from build123d import *

# Parameters (mm, degrees)
CROQUIS1_R              = 1.35
SALIENTE_EXTRUIR1_DEPTH = 10
CROQUIS2_W              = 7
CROQUIS2_H              = 28
SALIENTE_EXTRUIR2_DEPTH = 20
CROQUIS3_R              = 1.35
CORTAR_EXTRUIR1_DEPTH   = 15


with BuildPart() as part:
    # Croquis1 → Saliente-Extruir1 (new body)
    with BuildSketch(Plane(origin=(0, 0, 0), x_dir=(1, 0, 0), z_dir=(0, 1, 0))):
        Polygon((-20.25, -20), (-20.25, 8), (20.25, 8), (20.25, -20), (27.25, -20), (27.25, 20), (-27.25, 20), (-27.25, -20), align=None)
        with Locations(Location((-20.25, 15, 0), (0, 0, 270))):
            Circle(CROQUIS1_R, mode=Mode.SUBTRACT)
        with Locations(Location((20.25, 15, 0), (0, 0, 90))):
            Circle(CROQUIS1_R, mode=Mode.SUBTRACT)
    extrude(amount=SALIENTE_EXTRUIR1_DEPTH)

    # Croquis2 → Saliente-Extruir2 (add)
    with BuildSketch(Plane(origin=(0, 0, 0), x_dir=(1, 0, 0), z_dir=(0, 1, 0))):
        with Locations((-23.75, -6)):
            Rectangle(CROQUIS2_W, CROQUIS2_H)
        with Locations((23.75, -6)):
            Rectangle(CROQUIS2_W, CROQUIS2_H)
    extrude(amount=SALIENTE_EXTRUIR2_DEPTH)

    # Croquis3 → Cortar-Extruir1 (cut)
    with BuildSketch(Plane.XY.offset(20)):
        with Locations((-24.75, 15.612517806)):
            Circle(CROQUIS3_R)
        with Locations((-24.75, 4.5)):
            Circle(CROQUIS3_R)
        with Locations(Location((24.75, 4.5, 0), (0, 0, 180))):
            Circle(CROQUIS3_R)
        with Locations(Location((24.75, 15.612517806, 0), (0, 0, 180))):
            Circle(CROQUIS3_R)
    extrude(amount=-CORTAR_EXTRUIR1_DEPTH, mode=Mode.SUBTRACT)


solid = part.part
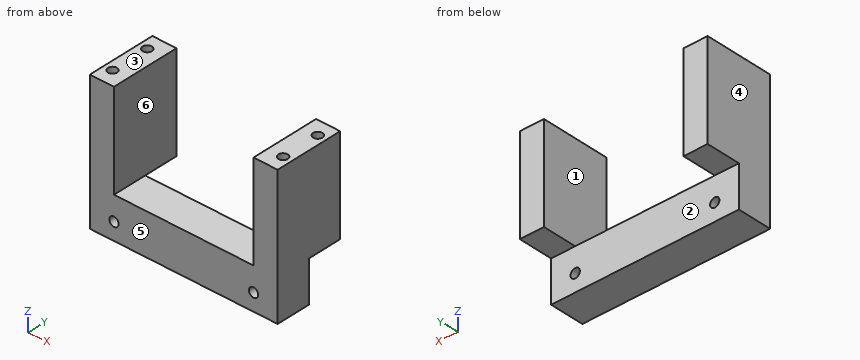
Build history of the part. All positions in model axes, mm. Face numbers are marked on the shaded views. A direction names the side the tool comes from. Coordinates: 2 decimals unless noted, no trailing zeros. Order: outer loops, then holes, each group sorted by start corner. A loop starts at its lowest first (then second) coordinate and runs counter-clockwise, first axis right, second up. Notation, with made-up numbers: (-38, 51) - (4, 51) arc R25 cw to (4, 77) - close; hole circle Ø2 at (18, 20.5). An arc over 180 degrees is marked (long way). Put each result on its own line as item: value.
1. Pull direction X, two halves, no side cores. Call the marked faces 4, 5 and 6: pulls with the +X half, pulls with the -X half, needs draft (parallel to the pull), parting line crosses it, or undercut.
Answer sheet:
face 4: pulls with the -X half
face 5: needs draft
face 6: undercut
2. Saw through at A-A (y = 2.25). Write the cut outline in (x, z).
Answer sheet:
outline: (-27.25, -20) - (27.25, -20) - (27.25, 20) - (20.25, 20) - (20.25, -8) - (-20.25, -8) - (-20.25, 20) - (-27.25, 20) - close; hole circle Ø2.7 at (-20.25, -15); hole circle Ø2.7 at (20.25, -15)
3. Saw through at B-B (z = -2). Write the cut outline in (x, y).
Answer sheet:
outline: (-27.25, 0) - (-20.25, 0) - (-20.25, 20) - (-27.25, 20) - close; (20.25, 0) - (27.25, 0) - (27.25, 20) - (20.25, 20) - close
4. Tool access for the marked faces 1, 2 and 3: list every direction of +Z, -Z, +X, -X, +Y, -Y with a clear straight run to the whole face (end or side of a thin tool).
Answer sheet:
face 1: +Z, +Y, -Y
face 2: -Z, +X, -X, +Y
face 3: +Z, +X, -X, +Y, -Y
5. Probe line 1 along Y through (x, z) = (24.75, 11.5); line 2 along X through (y, z) = (2, -4); line 3 along X through (y, z) = (15.5, 8.5). List the from-to ranges inside material, lowest first. Write a range as [from, to].
Answer sheet:
line 1: y = [0, 3.15], [5.85, 14.26], [16.96, 20]
line 2: x = [-27.25, -20.25], [20.25, 27.25]
line 3: x = [-27.25, -26.1], [-23.4, -20.25], [20.25, 23.4], [26.1, 27.25]
6. Drop flat-ended pins along their axis: P1, Ø3, axis at x = -9.5, y = 3.5, coming from the +Z side; P2, Ø0.8, axis at x = -24.5, y = 15.5, coming from the +Z side; P3, Ø2, axis at x = -24, y = 16.5, coming from the -Z side; P4, Ø2.5, axis at x = -20.25, z = -15, coming from the +Y side. Give the stop position or say it passes through.
Answer sheet:
P1: stops at z = -8
P2: stops at z = 5
P3: stops at z = -8
P4: passes through
7. Saw through at D-D (x = 19.5). Write the cut outline in (y, z).
Answer sheet:
outline: (0, -20) - (10, -20) - (10, -16.12) - (0, -16.12) - close; (0, -13.88) - (10, -13.88) - (10, -8) - (0, -8) - close
8. Saw through at C-C (z = 17.5). Write the cut outline in (x, y), and give its area (3 significant figures).
Answer sheet:
outline: (-27.25, 0) - (-20.25, 0) - (-20.25, 20) - (-27.25, 20) - close; (20.25, 0) - (27.25, 0) - (27.25, 20) - (20.25, 20) - close; hole circle Ø2.7 at (-24.75, 4.5); hole circle Ø2.7 at (-24.75, 15.61); hole circle Ø2.7 at (24.75, 4.5); hole circle Ø2.7 at (24.75, 15.61)
area: 257 mm^2
